Model file for the job. Use its own axes, mm. Face numbers are marked on the shaded views. A direction names the side the tool comes from. Round coordinates to 2 decimals unless told otherwise and drop trailing zeros. Order: outer loops, then holes, each group sorted by start corner. A loop starts at its lowest first (then second) coordinate and runs counter-clockwise, first axis right, second up. Notation, with made-up numbers: M -40,33.25 L -19,33.25 A24 ccw -19,48.25 Z; hole C -39,78.5 d1. An arc over 180 degrees is marked long. Return JSON: item names as keys, results as strings. Group by question number.
Item 1: Pull direction X, two halves, no side cores. Call the marked faces 1, 2 and 3: pulls with the +X half, pulls with the -X half, needs draft (parallel to the pull), parting line crosses it, or undercut.
Item 2: Probe line 1 along X through (y, z) = (15, -28.5); line 2 along X through (y, z) = (13.25, -24); line 3 along Y through (x, z) = (4.75, -26). List the from-to ranges inside material, lowest first.
Item 3: Pin check, flat tips, straight feed: pin 1 Ø6 at (x, y) = (15.5, 8.5) entering from -Z; pin 2 Ø10 at (x, z) = (3, -16) entering from -Y; pin 3 Ø5 at (x, z) = (24.5, -28) entering from +Y. Stop position of each tip, or through.
Item 4: Which spindle directions (+Z, -Z, +X, -X, +Y, -Y) get a long thin tool onto all of the face, cutting with end or side? Do the marked faces 4, 5 and 6. Say none if no direction does.
Item 5: Slice it at B-B on y = 7.5. Write the cut outline in (x, z).
Item 6: Slice it at C-C on z = -27.5. Give the number of separate pieces and of enclosed holes in the cut face, then the cut area to 3 significant figures.
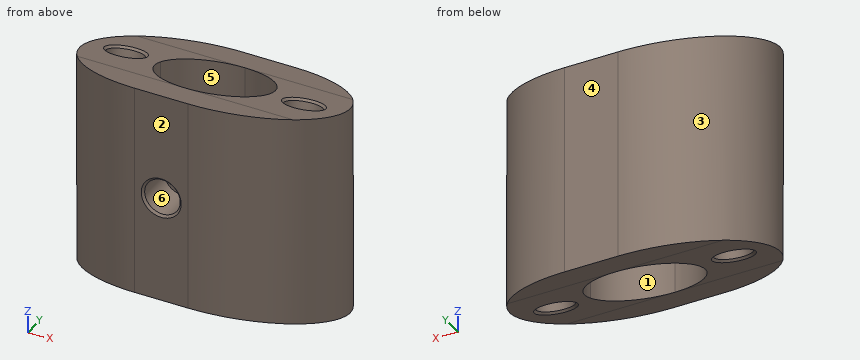
Autodesk Inventor part; units mm, degrees
ref_plane "YZ Plane" through (0, 0, 0) normal (1, 0, 0) x (0, 1, 0)
ref_plane "XZ Plane" through (0, 0, 0) normal (0, 1, 0) x (-1, 0, 0)
ref_plane "XY Plane" through (0, 0, 0) normal (0, 0, 1) x (1, 0, 0)
sketch "Sketch1" plane through (0, 0, 0) normal (1, 0, 0) x (0, 1, 0)
  line L0 (0, 0) -> (35.2385, -12.8258) construction
  line L1 (0, 0) -> (37.5, 0) construction
  line L2 (35.2385, -12.8258) -> (34.5544, -14.7051) construction
  line L3 (34.5544, -14.7051) -> (-0.684, -1.8794) construction
  line L4 (-0.684, -1.8794) -> (0, 0) construction
  line L5 (34.5544, -14.7051) -> (26.8932, -35.7543) construction
  line L6 (26.8932, -35.7543) -> (-8.3453, -22.9285) construction
  line L7 (-8.3453, -22.9285) -> (-9.0293, -24.8079) construction
  line L8 (-9.0293, -24.8079) -> (26.2091, -37.6336) construction
  line L9 (26.2091, -37.6336) -> (26.8932, -35.7543) construction
  line L10 (16.9352, -8.2923) -> (8.6633, -29.1191) construction
  line L11 (12.7992, 23.1416) -> (12.7992, -60.5529) construction
  line L12 (6.7992, 23.1416) -> (6.7992, -60.5529) construction
  line L13 (18.7992, 23.1416) -> (18.7992, -60.5529) construction
  line L14 (12.7992, -4.6585) -> (23.6057, -8.5918) construction
  line L15 (23.6057, -8.5918) -> (14.5764, -33.3997) construction
  line L16 (12.7992, -4.6585) -> (1.9928, -0.7253) construction
  line L17 (1.9928, -0.7253) -> (-7.0366, -25.5332) construction
  line L18 (1.7992, 23.1416) -> (1.7992, -60.5529)
  line L19 (23.7992, 23.1416) -> (23.7992, -60.5529)
  line L20 (18.9242, 23.1416) -> (18.9242, -60.5529)
  line L21 (6.6742, 23.1416) -> (6.6742, -60.5529)
  line L22 (1.7992, -2.7832) -> (6.6742, -4.5576)
  line L23 (1.7992, -26.6208) -> (6.6742, -28.3952)
  line L24 (23.7992, -34.6282) -> (18.9242, -32.8538)
  line L25 (23.7992, -10.7906) -> (18.9242, -9.0162)
  point P0 (12.7992, -18.7057)
  dimension "d1" = 37.5
  dimension "d2" = 20
  dimension "d3" = 2
  dimension "d4" = 22.4
  dimension "d5" = 37.5
  dimension "d6" = 2
  dimension "d7" = 6
  dimension "d8" = 6
  dimension "d9" = 11.5
  dimension "d10" = 11.5
  dimension "d13" = 11
  dimension "d14" = 11
  dimension "d15" = 4.875
  dimension "d16" = 4.875
extrude "Extrusion1" add sketch "Sketch1" along normal blind 28
sketch "Sketch2" plane through (28, 0, 0) normal (1, 0, 0) x (0, 0, -1)
  line L0 (28.3952, 6.6742) -> (4.5576, 6.6742)
  line L1 (9.0162, 18.9242) -> (32.8538, 18.9242)
  line L2 (4.5576, 6.6742) -> (9.0162, 18.9242)
  line L3 (9.0162, 18.9242) -> (32.8538, 18.9242)
  line L4 (32.8538, 18.9242) -> (28.3952, 6.6742)
  line L5 (28.3952, 6.6742) -> (4.5576, 6.6742)
  point P0 (0, 0)
  point P1 (28.3952, 6.6742)
extrude "Extrusion2" add sketch "Sketch2" against normal blind 7.875
sketch "Sketch3" plane through (0, 0, 0) normal (-1, 0, 0) x (0, 0, 1)
  line L0 (-9.0162, 18.9242) -> (-32.8538, 18.9242)
  line L1 (-26.6208, 1.7992) -> (-28.3952, 6.6742)
  line L2 (-32.8538, 18.9242) -> (-28.3952, 6.6742)
  line L3 (-28.3952, 6.6742) -> (-4.5576, 6.6742)
  line L4 (-4.5576, 6.6742) -> (-9.0162, 18.9242)
  line L5 (-9.0162, 18.9242) -> (-32.8538, 18.9242)
  point P0 (0, 0)
  point P1 (-9.0162, 18.9242)
extrude "Extrusion3" add sketch "Sketch3" against normal blind 7.875
fillet "Fillet1" radius 6.125 4 edges at (7.875, 6.6742, -16.4764) (20.125, 6.6742, -16.4764) (20.125, 18.9242, -20.935) (7.875, 18.9242, -20.935)
fillet "Fillet2" radius 11 4 edges at (0, 23.7992, -22.7094) (0, 1.7992, -14.702) (28, 1.7992, -14.702) (28, 23.7992, -22.7094)
sketch "Sketch4" plane through (11, 23.7992, -10.7906) normal (0, 0.3420201, 0.9396926) x (1, 0, 0)
  ellipse E0 centre (3, -11.706) end of major axis (3, -18.224) minor radius 6.125 construction
  circle A0 centre (3, -11.706) radius 10 construction
  circle A1 centre (-7, -11.706) radius 2
  circle A2 centre (13, -11.706) radius 2
  point P0 (-11, -26.0546)
  dimension "d25" = 20
  dimension "d26" = 4
  dimension "d27" = 4
extrude "Extrusion4" cut sketch "Sketch4" against normal blind 8
sketch "Sketch5" plane through (17, 1.7992, -26.6208) normal (0, -0.3420201, -0.9396926) x (-1, 0, 0)
  ellipse E0 centre (3, 11.706) end of major axis (3, 18.224) minor radius 6.125
  circle A0 centre (3, 11.706) radius 10 construction
  circle A1 centre (-7, 11.706) radius 2
  circle A2 centre (13, 11.706) radius 2
  point P0 (17, -10.7956)
  dimension "d30" = 20
  dimension "d31" = 4
  dimension "d32" = 4
extrude "Extrusion5" cut sketch "Sketch5" against normal blind 8 contours A1 | A2
sketch "Sketch6" plane through (11, 1.7992, -2.7832) normal (0, -1, 0) x (1, 0, 0)
  line L0 (0, -23.8376) -> (0, 0)
  line L1 (0, -11.9188) -> (6, -11.9188) construction
  line L2 (6, 0) -> (6, -23.8376)
  circle A0 centre (3, -11.9188) radius 2
  point P0 (-11, 2.7832)
  dimension "d35" = 4
extrude "Extrusion6" cut sketch "Sketch6" against normal blind 4.25
chamfer "Chamfer1" distance 0.25 angle 45 5 edges at (12, 1.7992, -14.702) (6, 12.7992, -30.6245) (26, 12.7992, -30.6245) (22, 12.7992, -6.7869) (2, 12.7992, -6.7869)
properties part number "Leg_Loadpipe_Mount" material "Nylon 6/6"
Output values:
{
 "1": {"face 1": "undercut", "face 2": "needs draft", "face 3": "pulls with the -X half"},
 "2": {"line 1": "0.22 to 2.52, 5.48 to 8.28, 19.72 to 22.52, 25.48 to 27.78", "line 2": "0.01 to 3.22, 4.78 to 7.89, 20.11 to 23.22, 24.78 to 27.99", "line 3": "3.75 to 12.51, 16.46 to 21.85"},
 "3": {"pin 1": "z = -29.11", "pin 2": "y = 2.22", "pin 3": "y = 22.6"},
 "4": {"face 4": "+Z, -Z, +X, -X, +Y", "face 5": "+Z, -Z", "face 6": "-Y"},
 "5": {"outline": "M 1.36,-28.7 L 10.93,-28.7 L 10.93,-4.86 L 1.36,-4.86 Z; M 17.07,-28.7 L 26.64,-28.7 L 26.64,-4.86 L 17.07,-4.86 Z"},
 "6": {"separate pieces": "1", "enclosed holes": "3", "area": "330 mm²"}
}
